Check sheet for the modelled part. Datum: model origin and axes. Units: mm. A direction names the side the tool comes from. Round coordinates to 2 decimals unless told otherwise and drop trailing zeros. Order: outer loops, then holes, each group sorted by start corner. A loop starts at its lowest first (then second) coordinate and runs counter-clockwise, first axis right, second up. Notation, with made-up numbers: (-32, 23.5) -> (-18, 23.5) arc R11 cw to (-18, 43.5) -> close; hole circle Ø11 at (72.25, -25). An arc over 180 degrees is marked (long way). Answer in a Markdown table with one row per item. Add a question column.
1. Access from +Z, -Z, +X, -X, +Y, -Y to the whole of each face (thin tool, end or side, straight path). Record for faces 4 (the flat face through (-27.009, -4.383, 47.856)), 5 (the flat face through (1, -10.16, -1)).
2. Material ranges on L1, parallel to Y at x = 41, z = 25; L2, parallel to X at y = -11, z = -10.5; L3, parallel to Z at x = 2.5, y = -12, recorded low to high. Write a range as from..to.
3. Sectioned sample at C-C, the plane y = -6.5. Record the boundary of the cut face in (x, z).
4. Sectioned sample at A-A, the plane z = -34. Record the boundary of the cut face in (x, y), then the cut area to 3 significant figures.
5. Draft check along X on faces 1 (the flat face through (57.3, -10.82, -7.47)), 2 (the flat face through (-27.776, -4.383, -56.448)), 3 (the flat face through (-25.086, -11.448, 44.529)). Enter one of: +X half, -X half, draft (parallel to the pull), parting line (faces both ways), or undercut.
6. Sectioned sample at B-B, the plane x = -13. Record the boundary of the cut face in (y, z), then the cut area to 3 significant figures.
7. Depth check by flat-ended pin: P1, Ø1.5, axis at x = 9, y = -3.5, coming from the +Z side; P2, Ø3, axis at x = 7, y = -4, coming from the +Z side; P3, Ø6, axis at x = -8.5, y = -9.5, coming from the +Z side. Enter the tip coordinate at first touch or a pass-through.
```python
from build123d import *

# Parameters (mm, degrees)
F1_DEPTH = 12.7
F2_SIZE  = 3.81
F3_DEPTH = 2.54


with BuildPart() as f1:
    # F0 (on Front) → F1 (new body)
    with BuildSketch(Plane.XZ):
        Polygon((59.229627, 26.558874), (0, 68.564124), (-54.784626, 26.558874), (-54.784626, -40.560622), (0, -72.786875), (59.229627, -40.560622), align=None)
    extrude(amount=F1_DEPTH)

    # F2
    f2_edges = [f1.edges().sort_by_distance(p)[0] for p in [
        (59.229627, -12.7, -7.000874),
        (29.614814, -12.7, 47.561499),
        (-27.392313, -12.7, 47.561499),
        (-54.784626, -12.7, -7.000874),
        (-27.392313, -12.7, -56.673748),
        (29.614814, -12.7, -56.673748),
    ]]
    chamfer(f2_edges, length=F2_SIZE)

    # F1_face (on face) → F3 (cut)
    with BuildSketch(Plane(origin=(1.953457, -12.7, -4.300965), x_dir=(1, 0, 0), z_dir=(0, -1, 0))):
        Polygon((53.46617, -33.995203), (53.46617, 28.890993), (-1.865273, 68.131678), (-52.928083, 28.980071), (-52.928083, -34.080543), (-1.880286, -64.108661), align=None)
    extrude(amount=-F3_DEPTH, mode=Mode.SUBTRACT)


solid = f1.part
```
Answer key:
| question | item | result |
|---|---|---|
| 1 | face 4 | +Z, -X, +Y, -Y |
| 1 | face 5 | -Y |
| 2 | L1 | y = -10.16..0 |
| 2 | L2 | x = -52.67..-50.97, 55.42..57.12 |
| 2 | L3 | z = -67.89..-67.09, 62.12..62.98 |
| 3 | outline | (-54.78, -40.56) -> (0, -72.79) -> (59.23, -40.56) -> (59.23, 26.56) -> (0, 68.56) -> (-54.78, 26.56) -> close |
| 4 | outline | (-54.78, -8.89) -> (-50.97, -12.7) -> (-50.97, -10.16) -> (55.42, -10.16) -> (55.42, -12.7) -> (59.23, -8.89) -> (59.23, 0) -> (-54.78, 0) -> close |
| 4 | area | 1,160 mm² |
| 5 | face 1 | +X half |
| 5 | face 2 | -X half |
| 5 | face 3 | undercut |
| 6 | outline | (-12.7, -60.72) -> (-8.89, -65.14) -> (0, -65.14) -> (0, 58.6) -> (-8.89, 58.6) -> (-12.7, 53.8) -> (-10.16, 53.8) -> (-10.16, -60.72) -> close |
| 6 | area | 1,260 mm² |
| 7 | P1 | stops at z = 62.71 |
| 7 | P2 | stops at z = 64.66 |
| 7 | P3 | stops at z = 64.3 |
